from build123d import *

# Parameters (mm, degrees)
SKETCH1_W          = 30
SKETCH1_H          = 30
EXTRUDE1_DEPTH     = 10
SKETCH2_W          = 21
SKETCH2_H          = 21
EXTRUDE2_DEPTH     = 2
SKETCH3_R          = 7.5
EXTRUDE3_DEPTH     = 8
SKETCH4_R          = 6
EXTRUDE4_DEPTH     = 5.5
SKETCH5_R          = 7
EXTRUDE5_DEPTH     = 3
SKETCH6_R          = 5
CUT_EXTRUDE1_DEPTH = 3
CHAMFER1_SIZE      = 3
FILLET1_R          = 1
FILLET2_R          = 2


with BuildPart() as part:
    # Sketch1 → Extrude1 (new body)
    with BuildSketch(Plane.XY):
        Rectangle(SKETCH1_W, SKETCH1_H)
    extrude(amount=EXTRUDE1_DEPTH)

    # Sketch2 → Extrude2 (add)
    with BuildSketch(Plane.XY.offset(10)):
        Rectangle(SKETCH2_W, SKETCH2_H)
    extrude(amount=EXTRUDE2_DEPTH)

    # Sketch3 → Extrude3 (add)
    with BuildSketch(Plane.XY.offset(12)):
        with Locations(Location((0, 0, 0), (0, 0, 180))):
            Circle(SKETCH3_R)
    extrude(amount=EXTRUDE3_DEPTH)

    # Sketch4 → Extrude4 (add)
    with BuildSketch(Plane.XY.offset(20)):
        Circle(SKETCH4_R)
    extrude(amount=EXTRUDE4_DEPTH)

    # Sketch5 → Extrude5 (add)
    with BuildSketch(Plane.XY.offset(25.5)):
        Circle(SKETCH5_R)
    extrude(amount=EXTRUDE5_DEPTH)

    # Sketch6 → Cut-Extrude1 (cut)
    with BuildSketch(Plane.XY.offset(28.5)):
        Circle(SKETCH6_R)
    extrude(amount=-CUT_EXTRUDE1_DEPTH, mode=Mode.SUBTRACT)

    # Chamfer1
    chamfer1_edges = [part.edges().sort_by_distance(p)[0] for p in [
        (-5, 0, 25.5),
    ]]
    chamfer(chamfer1_edges, length=CHAMFER1_SIZE - 0.0001)  # a hair under: the kernel refuses the full size

    # Sketch8 → Revolve1 (revolve)
    with BuildSketch(Plane(origin=(0, 0, 0), x_dir=(0, 0, -1), z_dir=(1, 0, 0)), mode=Mode.PRIVATE) as revolve1_sk:
        with BuildLine():
            Line((-25.5, 0), (-25.5, 6))
            add(Edge.make_bspline(
                [(-28.5, 0), (-28.329286333, 3.962436502), (-27.079878372, 4.87576544), (-25.5, 6)],
                knots=[0, 0, 0, 0, 1, 1, 1, 1], degree=3))
            Line((-28.5, 0), (-25.5, 0))
        make_face()
    revolve(revolve1_sk.sketch.rotate(Axis((0, 0, 28.5), (0, 0, -1)), 90), axis=Axis((0, 0, 28.5), (0, 0, -1)))

    # Fillet1
    fillet1_edges = [part.edges().sort_by_distance(p)[0] for p in [
        (15, 0, 10),
        (0, 15, 10),
        (-15, 0, 10),
        (0, -15, 10),
        (-15, 15, 5),
        (15, 15, 5),
        (15, -15, 5),
        (-15, -15, 5),
    ]]
    fillet(fillet1_edges, radius=FILLET1_R)

    # Fillet2
    fillet2_edges = [part.edges().sort_by_distance(p)[0] for p in [
        (0, -10.5, 12),
        (10.5, 0, 12),
        (0, 10.5, 12),
        (-10.5, 0, 12),
    ]]
    fillet(fillet2_edges, radius=FILLET2_R - 0.0001)  # a hair under: the kernel refuses the full size


solid = part.part
Geometry: final body of the model. Coordinates: model frame, mm. A direction names the side the tool comes from. Give positions to 0.01 mm unless a question says otherwise; leave off trailing zeros. Write each loop counter-clockwise with the first axis right and the second up, starting at its lowest first coordinate (ties: lowest second). Pieces come first, ordered by that corner, then holes.
(1) Cut plane A-A, the plane y = -12. Return loops of the section in (x, z), then the cut area to 3 significant figures.
(2) Access query for faces 1 (the cylindrical face through (-4.032, -6.324, 15.944)), 2 (the flat face through (6, 2, 25.5)), 3 (the cylindrical face through (14.699, 14.715, 4.563)). Directions: +Z, -Z, +X, -X, +Y, -Y. A direction counts if a zero-diameter tool reaches every point of the face in a straight line with its end or side. Return the directions, or none.
(3) Ray query, line 1 (Z direction, x = -0.25, y = 6.5); line 2 (Z direction, x = 4.25, y = 13.25); line 3 (Z direction, x = 0.5, y = 7.75). Return the intervals inside material, ascending.
(4) First-contact query: P1, Ø1, axis at x = -6.5, z = 19.5, coming from the -Y side; P2, Ø3, axis at y = 7.5, z = 20.5, coming from the -X side; P3, Ø10, axis at y = 4.5, z = 19, coming from the +X side. Flat tips, straight axial feed; report the tip coordinate or a pass-through.
(5) Cut plane C-C, the plane z = 16.5. Return loops of the section in (x, y).
Values follow:
1. outline: (-15, 0) - (15, 0) - (15, 9) arc R1 ccw to (14, 10) - (-14, 10) arc R1 ccw to (-15, 9) - close
1. area: 300 mm2
2. face 1: +Z
2. face 2: none
2. face 3: +Z, -Z, +X, +Y
3. line 1: z = 0 to 20, 25.5 to 28.5
3. line 2: z = 0 to 10
3. line 3: z = 0 to 12
4. P1: stops at y = -4.5
4. P2: stops at x = -4.38
4. P3: stops at x = 7.5
5. outline: circle Ø15 at (0, 0)
